Source: CAD feature listing. Evaluate the final solid. Frame: model axes, mm. A direction names the side the tool comes from. Give positions to 0.01 mm unless a question says otherwise; leave off trailing zeros. Write each loop counter-clockwise with the first axis right and the second up, starting at its lowest first coordinate (ties: lowest second). Pieces come first, ordered by that corner, then holes. Notation, with made-up numbers: M -36.5,25.25 L -15.5,25.25 A12 ccw -15.5,32.25 Z; hole C 70,75.25 d3. An arc over 180 degrees is marked long. Use CSV: the item, a comma, the result in double quotes. Start each with the question number.
from build123d import *

# Parameters (mm, degrees)
SKETCH1_R           = 1.5
BOSS_EXTRUDE1_DEPTH = 2
CUT_EXTRUDE1_DEPTH  = 81.447719073
SKETCH3_R           = 5
CUT_EXTRUDE2_DEPTH  = 81.447719073


with BuildPart() as part:
    # Sketch1 → Boss-Extrude1 (new body)
    with BuildSketch(Plane(origin=(0, 0, 0), x_dir=(1, 0, 0), z_dir=(0, 1, 0))):
        with BuildLine():
            ThreePointArc((-34.963763955, -42.691134729), (-29.856641946, -52.293165337), (-19.005975188, -51.555115262))
            ThreePointArc((-19.005975188, -51.555115262), (0.154155805, -47.566469585), (19.272821809, -51.749354259))
            ThreePointArc((19.272821809, -51.749354259), (30.141985248, -52.127472163), (34.928148513, -42.361494065))
            ThreePointArc((34.928148513, -42.361494065), (41.005634123, -23.636153056), (54.236585765, -9.05821953))
            ThreePointArc((54.236585765, -9.05821953), (59.998627194, 0.165693174), (53.934123701, 9.193621197))
            ThreePointArc((53.934123701, 9.193621197), (41.034184142, 23.742001216), (35.148040543, 42.273518027))
            ThreePointArc((35.148040543, 42.273518027), (30.040918534, 51.875548635), (19.190251776, 51.13749856))
            ThreePointArc((19.190251776, 51.13749856), (-0.053987233, 47.109599988), (-19.274467503, 51.249387444))
            ThreePointArc((-19.274467503, 51.249387444), (-30.143630941, 51.627505348), (-34.929794206, 41.86152725))
            ThreePointArc((-34.929794206, 41.86152725), (-41.05559122, 23.274044232), (-54.237408611, 8.808236123))
            ThreePointArc((-54.237408611, 8.808236123), (-59.999450041, -0.415676581), (-53.934946548, -9.443604604))
            ThreePointArc((-53.934946548, -9.443604604), (-40.900612569, -24.042441945), (-34.963763955, -42.691134729))
        make_face()
        with Locations(Location((50, 0, 0), (0, 0, 90))):
            Circle(SKETCH1_R, mode=Mode.SUBTRACT)
        with Locations(Location((24.999177153, -43.551253597, 0), (0, 0, 90))):
            Circle(SKETCH1_R, mode=Mode.SUBTRACT)
        with Locations(Location((25.185099435, 43.133636895, 0), (0, 0, 90))):
            Circle(SKETCH1_R, mode=Mode.SUBTRACT)
        with Locations(Location((-25.000822847, -43.551253597, 0), (0, 0, 90))):
            Circle(SKETCH1_R, mode=Mode.SUBTRACT)
        with Locations(Location((-50.000822847, -0.249983407, 0), (0, 0, 90))):
            Circle(SKETCH1_R, mode=Mode.SUBTRACT)
        with Locations(Location((-25.000822847, 43.051286782, 0), (0, 0, 90))):
            Circle(SKETCH1_R, mode=Mode.SUBTRACT)
    extrude(amount=-BOSS_EXTRUDE1_DEPTH)

    # Sketch2 → Cut-Extrude1 (cut, through all)
    with BuildSketch(Plane(origin=(0, 0, 0), x_dir=(1, 0, 0), z_dir=(0, 1, 0))):
        with BuildLine():
            Line((-20.75, 25), (-20.75, -25))
            ThreePointArc((-20.75, -25), (-25, -29.25), (-29.25, -25))
            Line((-29.25, -25), (-29.25, 25))
            ThreePointArc((-29.25, 25), (-25, 29.25), (-20.75, 25))
        make_face()
        with BuildLine():
            Line((20.75, 25), (20.75, -25))
            ThreePointArc((20.75, -25), (25, -29.25), (29.25, -25))
            Line((29.25, -25), (29.25, 25))
            ThreePointArc((29.25, 25), (25, 29.25), (20.75, 25))
        make_face()
    extrude(amount=-CUT_EXTRUDE1_DEPTH, mode=Mode.SUBTRACT)

    # Sketch3 → Cut-Extrude2 (cut, through all)
    with BuildSketch(Plane(origin=(0, 0, 0), x_dir=(1, 0, 0), z_dir=(0, 1, 0))):
        with Locations(Location((0, 0, 0), (0, 0, 270))):
            Circle(SKETCH3_R)
    extrude(amount=-CUT_EXTRUDE2_DEPTH, mode=Mode.SUBTRACT)


solid = part.part
1. First-contact query: pin 1 (1 mm diameter, centred on y = -2, z = -7.5, fed in from +X); pin 2 (0.6 mm diameter, centred on y = -1, z = 1, fed in from +X); pin 3 (1 mm diameter, centred on y = -1, z = 8.5, fed in from -X). Flat tips, straight axial feed; report the tip coordinate or a pass-through.
2. Section B-B on y = -1.35. Give the number of separate pieces and of enclosed holes in the cut face, then the cut area to 3 significant figures.
3. Access query for faces 1 (the cylindrical face through (60, -1, 0)), 2 (the cylindrical face through (-25.09, -0.99, -29.25)). Directions: +Z, -Z, +X, -X, +Y, -Y. A direction counts if a zero-diameter tool reaches every point of the face in a straight line with its end or side. Return the directions, or none.
4. Section A-A on x = -3.5. Return loops of the section in (y, z).
5. Pull-direction query (Z, two-part tool) for faces 3 (the cylindrical face through (0.22, -0.99, -47.11)), 4 (the cylindrical face through (-51.488, -0.986, 0.445)), 5 (the cylindrical face through (-41.04, -0.99, 23.8)), 6 (the flat face through (-1, -2, 11)); classes: released by +Z, released by -Z, zero draft, split by the parting line, or undercut.
6. Section D-D on x = 50. Return loops of the section in (y, z), then the cut area to 3 significant figures.
7. Line query: probe 1 along X at (y, z) = (-0.65, -14.5); probe 2 along X at (y, z) = (-1.2, 22); probe 3 along X at (y, z) = (-0.55, 3.5). Output: solid intervals per line, ascending.
8. Section C-C on z = -11.5. Return loops of the section in (x, y), then the cut area to 3 significant figures.
Resolved:
1,pin 1,"stops at x = 57.14"
1,pin 2,"stops at x = 59.98"
1,pin 3,"stops at x = -56.32"
2,separate pieces,"1"
2,enclosed holes,"9"
2,area,"7,620 mm2"
3,face 1,"+X, +Y, -Y"
3,face 2,"+Y, -Y"
4,outline,"M -2,-47.25 L 0,-47.25 L 0,-3.57 L -2,-3.57 Z; M -2,3.57 L 0,3.57 L 0,47.69 L -2,47.69 Z"
5,face 3,"released by -Z"
5,face 4,"undercut"
5,face 5,"released by +Z"
5,face 6,"zero draft"
6,outline,"M -2,-12.45 L 0,-12.45 L 0,-1.5 L -2,-1.5 Z; M -2,1.5 L 0,1.5 L 0,12.49 L -2,12.49 Z"
6,area,"43.9 mm2"
7,probe 1,"x = -47.67 to -29.25, -20.75 to 20.75, 29.25 to 47.91"
7,probe 2,"x = -42.14 to -29.25, -20.75 to 20.75, 29.25 to 42"
7,probe 3,"x = -59.46 to -29.25, -20.75 to -3.57, 3.57 to 20.75, 29.25 to 59.37"
8,outline,"M -50.82,-2 L -29.25,-2 L -29.25,0 L -50.82,0 Z; M -20.75,-2 L 20.75,-2 L 20.75,0 L -20.75,0 Z; M 29.25,-2 L 51.06,-2 L 51.06,0 L 29.25,0 Z"
8,area,"170 mm2"
